```python
from build123d import *

# Parameters (mm, degrees)
SKETCH2_R           = 63.5
BOSS_EXTRUDE1_DEPTH = 190.5
SKETCH3_R           = 50.8
BOSS_EXTRUDE2_DEPTH = 101.6
SKETCH4_R           = 101.6
BOSS_EXTRUDE3_DEPTH = 63.5
FILLET1_R           = 2.54
FILLET2_R           = 2.54


with BuildPart() as part:
    # Sketch2 → Boss-Extrude1 (new, symmetric)
    with BuildSketch(Plane(origin=(0, 0, 0), x_dir=(0, 0, -1), z_dir=(1, 0, 0))):
        Circle(SKETCH2_R)
    extrude(amount=BOSS_EXTRUDE1_DEPTH, both=True)

    # Sketch3 → Boss-Extrude2 (add)
    with BuildSketch(Plane.ZY.offset(190.5)):
        Circle(SKETCH3_R)
    extrude(amount=BOSS_EXTRUDE2_DEPTH)

    # Sketch4 → Boss-Extrude3 (add)
    with BuildSketch(Plane(origin=(190.5, 0, 0), x_dir=(0, 0, -1), z_dir=(1, 0, 0))):
        Circle(SKETCH4_R)
    extrude(amount=BOSS_EXTRUDE3_DEPTH)

    # Fillet1
    fillet1_edges = [part.edges().sort_by_distance(p)[0] for p in [
        (254, 0, 101.6),
        (190.5, 0, 101.6),
    ]]
    fillet(fillet1_edges, radius=FILLET1_R)

    # Fillet2
    fillet2_edges = [part.edges().sort_by_distance(p)[0] for p in [
        (-190.5, 0, 63.5),
        (-292.1, 0, -50.8),
    ]]
    fillet(fillet2_edges, radius=FILLET2_R)


solid = part.part
```
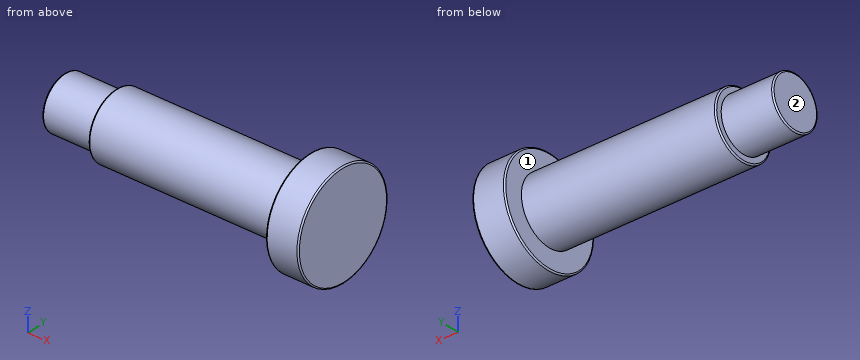
Can you work these out from the model? Positions are in its coordinate system, mm. Face numbers are marked on the shaded views. A direction names the side the tool comes from. Coordinates: 2 decimals unless noted, no trailing zeros. Loops run counter-clockwise (first coordinate to the right, second up) from the corner with the lowest first, then second, coordinate; pieces in that order, holes last.
1) Imagine slicing it at C-C on x = -153. List the corners of the cut face in (y, z) for me.
2) Imagine slicing it at A-A on z = 0. List the corners of the cut face in (x, y) for me.
3) I need wall thicknesses on probe 1 along X at (y, z) = (62, -62); probe 2 along X at (y, z) = (50.5, -17.5); probe 3 along Z at (x, y) = (7, 40.5). Which ranges of each line are inside material? Lowest first, please.
4) Imagine slicing it at D-D on x = -255.5. List the corners of the cut face in (y, z) for me.
5) For pin 1 (2 mm diameter, centred on y = 70.5, z = -60.5, fed in from -X); pin 2 (3 mm diameter, centred on x = -74, z = 14, fed in from +Y); pin 3 (4 mm diameter, centred on x = 147.5, z = 14, fed in from +Y), each with a flat end and sliding along its axis, tell me the tip position at first contact or that it passes through.
6) Which directions (+Z, -Z, +X, -X, +Y, -Y) give clear straight access to the entire face, cutting with the end or side of a thin tool? Please do the marked faces 1 and 2.
Completed:
1. outline: circle Ø127 at (0, 0)
2. outline: (-292.1, -48.26) arc R2.54 ccw to (-289.56, -50.8) - (-190.5, -50.8) - (-190.5, -60.96) arc R2.54 ccw to (-187.96, -63.5) - (190.5, -63.5) - (190.5, -99.06) arc R2.54 ccw to (193.04, -101.6) - (251.46, -101.6) arc R2.54 ccw to (254, -99.06) - (254, 99.06) arc R2.54 ccw to (251.46, 101.6) - (193.04, 101.6) arc R2.54 ccw to (190.5, 99.06) - (190.5, 63.5) - (-187.96, 63.5) arc R2.54 ccw to (-190.5, 60.96) - (-190.5, 50.8) - (-289.56, 50.8) arc R2.54 ccw to (-292.1, 48.26) - close
3. probe 1: x = 190.5 to 254
3. probe 2: x = -190.5 to 254
3. probe 3: z = -48.91 to 48.91
4. outline: circle Ø101.6 at (0, 0)
5. pin 1: stops at x = 190.5
5. pin 2: stops at y = 62.26
5. pin 3: stops at y = 62.36
6. face 1: -X
6. face 2: +Z, -Z, -X, +Y, -Y
